For this review, take the finished solid that the model builds, in its own axes (mm). Face numbers are marked on the shaded views. Round coordinates to 2 decimals unless told otherwise and drop trailing zeros. Order: outer loops, then holes, each group sorted by start corner. A loop starts at its lowest first (then second) coordinate and runs counter-clockwise, first axis right, second up. Notation, with made-up numbers: (52.25, -21) -> (61.25, -21) arc R30 ccw to (61.25, 2) -> close; hole circle Ø2 at (-10.5, -35). An arc over 180 degrees is marked (long way). Answer in a Markdown table with one row per item.
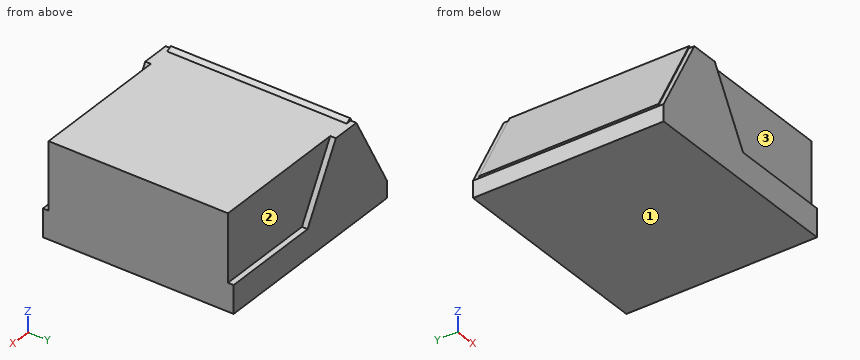
```python
from build123d import *

# Parameters (mm, degrees)
SKETCH_W     = 177.5
SKETCH_H     = 160
PAD_DEPTH    = 5
SKETCH001_W  = 5
SKETCH001_H  = 15
PAD001_DEPTH = 160
SKETCH002_W  = 5
SKETCH002_H  = 75
PAD002_DEPTH = 160
SKETCH003_W  = 20
SKETCH003_H  = 5
PAD003_DEPTH = 160
SKETCH004_W  = 120
SKETCH004_H  = 5
PAD004_DEPTH = 160
SKETCH005_W  = 160
SKETCH005_H  = 25
PAD005_DEPTH = 5
PAD006_DEPTH = 5
PAD007_DEPTH = 160
SKETCH008_W  = 125
SKETCH008_H  = 60
PAD008_DEPTH = 5
SKETCH009_W  = 5
SKETCH009_H  = 60
PAD009_DEPTH = 150
SKETCH010_W  = 5
SKETCH010_H  = 60
PAD010_DEPTH = 150
SKETCH011_W  = 115
SKETCH011_H  = 150
PAD011_DEPTH = 5


with BuildPart() as part:
    # Sketch → Pad (new body)
    with BuildSketch(Plane.XY):
        with Locations((31.25, 0)):
            Rectangle(SKETCH_W, SKETCH_H)
    extrude(amount=PAD_DEPTH)

    # Sketch001 (on Face3 of Pad) → Pad001 (join)
    with BuildSketch(Plane.XZ.offset(80)):
        with Locations((-60, 7.5)):
            Rectangle(SKETCH001_W, SKETCH001_H)
    extrude(amount=-PAD001_DEPTH)

    # Sketch002 (on Face3 of Pad001) → Pad002 (join)
    with BuildSketch(Plane.XZ.offset(80)):
        with Locations((-2.5, 42.5)):
            Rectangle(SKETCH002_W, SKETCH002_H)
    extrude(amount=-PAD002_DEPTH)

    # Sketch003 (on Face10 of Pad002) → Pad003 (join)
    with BuildSketch(Plane.XZ.offset(80)):
        with Locations((-10, 82.5)):
            Rectangle(SKETCH003_W, SKETCH003_H)
    extrude(amount=-PAD003_DEPTH)

    # Sketch004 (on Face3 of Pad003) → Pad004 (join)
    with BuildSketch(Plane.XZ.offset(80)):
        with Locations((60, 22.5)):
            Rectangle(SKETCH004_W, SKETCH004_H)
    extrude(amount=-PAD004_DEPTH)

    # Sketch005 (on Face28 of Pad004) → Pad005 (join)
    with BuildSketch(Plane.YZ.offset(120)):
        with Locations((0, 12.5)):
            Rectangle(SKETCH005_W, SKETCH005_H)
    extrude(amount=PAD005_DEPTH)

    # Sketch006 (on Face11 of Pad005) → Pad006 (join)
    with BuildSketch(Plane(origin=(0, 80, 0), x_dir=(-1, 0, 0), z_dir=(0, 1, 0))):
        Polygon((62.5, 15), (62.5, 0), (-125, 0), (-125, 25), (-34.641016, 25), (0, 85), (25, 85), align=None)
    pad006 = extrude(amount=PAD006_DEPTH)

    # Sketch007 (on Face14 of Pad006) → Pad007 (join)
    with BuildSketch(Plane.XZ.offset(80)):
        Polygon((-57.5, 15), (-20, 85), (-24.4074, 87.361107), (-61.9074, 17.361107), align=None)
    extrude(amount=-PAD007_DEPTH)

    # Mirrored: Pad006 across XZ
    add(pad006.mirror(Plane.XZ))

    # Sketch008 (on Face36 of Mirrored) → Pad008 (join)
    with BuildSketch(Plane(origin=(0, -80, 0), x_dir=(-1, 0, 0), z_dir=(0, 1, 0))):
        with Locations((-62.5, 55)):
            Rectangle(SKETCH008_W, SKETCH008_H)
    pad008 = extrude(amount=PAD008_DEPTH)

    # Sketch009 (on Face37 of Pad008) → Pad009 (join)
    with BuildSketch(Plane(origin=(0, -75, 0), x_dir=(-1, 0, 0), z_dir=(0, 1, 0))):
        with Locations((-122.5, 55)):
            Rectangle(SKETCH009_W, SKETCH009_H)
    extrude(amount=PAD009_DEPTH)

    # Sketch010 (on Face39 of Pad009) → Pad010 (join)
    with BuildSketch(Plane(origin=(0, -75, 0), x_dir=(-1, 0, 0), z_dir=(0, 1, 0))):
        with Locations((-2.5, 55)):
            Rectangle(SKETCH010_W, SKETCH010_H)
    extrude(amount=PAD010_DEPTH)

    # Mirrored001: Pad008 across XZ
    add(pad008.mirror(Plane.XZ))

    # Sketch011 (on Face30 of Mirrored001) → Pad011 (join)
    with BuildSketch(Plane.XY.offset(85)):
        with Locations((62.5, 0)):
            Rectangle(SKETCH011_W, SKETCH011_H)
    extrude(amount=-PAD011_DEPTH)


solid = part.part
```
Q1. Take a section at D-D, the plane z = 55.5. Write out the cut boundary in (x, y), then the cut area to 3 significant figures.
Answer key:
| item | result |
|---|---|
| outline | (-41.48, -80) -> (-40.8, -80) -> (-40.8, -85) -> (17.03, -85) -> (17.03, -80) -> (125, -80) -> (125, 80) -> (17.03, 80) -> (17.03, 85) -> (-40.8, 85) -> (-40.8, 80) -> (-41.48, 80) -> close; hole (-35.8, -80) -> (-5, -80) -> (-5, 80) -> (-35.8, 80) -> close; hole (5, -75) -> (120, -75) -> (120, 75) -> (5, 75) -> close |
| area | 5,040 mm^2 |
Q2. Clearance check with flat-ended pins moving along their axes: pin 1 Ø12.5 at (x, z) = (-48, 46.5) entering from +Y; pin 2 Ø8 at (x, y) = (73, -6) entering from +Z; pin 3 Ø1.5 at (y, z) = (30.5, 83) entering from -X; pin 4 Ø2.5 at (x, y) = (-59.5, 18.5) entering from +Z. State where each tip first meets the part, or that it passes through.
Answer key:
| item | result |
|---|---|
| pin 1 | stops at y = 85 |
| pin 2 | stops at z = 85 |
| pin 3 | stops at x = -27.15 |
| pin 4 | stops at z = 24.19 |
Q3. Take a section at C-C, the plane x = -15. Write out the cut boundary in (y, z).
Answer key:
| item | result |
|---|---|
| outline | (-85, 0) -> (85, 0) -> (85, 85) -> (-85, 85) -> close; hole (-80, 5) -> (80, 5) -> (80, 80) -> (-80, 80) -> close |
Q4. To check wall thickness, follow probe 1 along Z at (x, y) = (66, 29); probe 2 along X at (y, z) = (51.5, 6); probe 3 along Y at (x, z) = (46, 74). State the ranges of each line that lie inside material, in increasing order.
Answer key:
| item | result |
|---|---|
| probe 1 | z = 0 to 5, 20 to 25, 80 to 85 |
| probe 2 | x = -62.5 to -57.5, -5 to 0, 120 to 125 |
| probe 3 | y = -80 to -75, 75 to 80 |
Q5. The part is to be moulded in two halves that separate along Y. For the marked faces 1, 2 and 3, say which applies: +Y half, -Y half, draft (parallel to the pull), parting line (faces both ways), or undercut.
Answer key:
| item | result |
|---|---|
| face 1 | draft |
| face 2 | +Y half |
| face 3 | -Y half |
Q6. Take a section at B-B, the plane x = 84.5. Write out the cut boundary in (y, z), then the cut area to 3 significant figures.
Answer key:
| item | result |
|---|---|
| outline | (-85, 0) -> (85, 0) -> (85, 25) -> (80, 25) -> (80, 85) -> (-80, 85) -> (-80, 25) -> (-85, 25) -> close; hole (-80, 5) -> (80, 5) -> (80, 20) -> (-80, 20) -> close; hole (-75, 25) -> (75, 25) -> (75, 80) -> (-75, 80) -> close |
| area | 3,200 mm^2 |
